Build history of the part. All positions in model axes, mm. A direction names the side the tool comes from. Give positions to 0.01 mm unless a question says otherwise; leave off trailing zeros. Order: outer loops, then holes, each group sorted by start corner. A loop starts at its lowest first (then second) coordinate and runs counter-clockwise, first axis right, second up. Notation, with made-up numbers: (58.5, -12.5) -> (66.5, -12.5) arc R12 ccw to (66.5, 0.5) -> close; hole circle Ø2 at (69.5, -32.5). An arc over 180 degrees is marked (long way). Write item = value, one per line. Start each with the question number.
Autodesk Inventor part; units mm, degrees
ref_plane "YZ Plane" through (0, 0, 0) normal (1, 0, 0) x (0, 1, 0)
ref_plane "XZ Plane" through (0, 0, 0) normal (0, 1, 0) x (-1, 0, 0)
ref_plane "XY Plane" through (0, 0, 0) normal (0, 0, 1) x (1, 0, 0)
sketch "Sketch1" plane through (0, 0, 0) normal (0, 0, 1) x (1, 0, 0)
  line L0 (51, -45) -> (-51, -45)
  line L1 (-51, -45) -> (-51, 45)
  line L2 (-51, 45) -> (51, 45)
  line L3 (51, 45) -> (51, -45)
  line L4 (51, -45) -> (-51, 45) construction
  line L5 (-51, -45) -> (51, 45) construction
  line L6 (-22, 0) -> (22, 0) construction
  line L7 (-36, 35) -> (-8, 35)
  line L8 (-8, 35) -> (-8, -35)
  line L9 (-8, -35) -> (-36, -35)
  line L10 (-36, -35) -> (-36, 35)
  line L11 (-36, 35) -> (-8, -35) construction
  line L12 (-8, 35) -> (-36, -35) construction
  line L13 (36, 35) -> (8, 35)
  line L14 (8, 35) -> (8, -35)
  line L15 (8, -35) -> (36, -35)
  line L16 (36, -35) -> (36, 35)
  line L17 (36, 35) -> (8, -35) construction
  line L18 (8, 35) -> (36, -35) construction
  point P0 (0, 0)
  point P1 (0, 0)
  dimension "d0" = 16
  dimension "d1" = 28
  dimension "d2" = 28
  dimension "d3" = 70
  dimension "d4" = 10
  dimension "d5" = 15
extrude "Extrusion1" add sketch "Sketch1" along normal blind 19
sketch "Sketch2" plane through (51, -45, 0) normal (1, 0, 0) x (0, 0, -1)
  circle A0 centre (0, 45) radius 7
  point P0 (0, 45)
  dimension "d8" = 14
extrude "Extrusion2" cut sketch "Sketch2" against normal through all
sketch "Sketch3" plane through (51, -45, 19) normal (1, 0, 0) x (0, 0, -1)
  arc A0 (19, 52) -> (19, 38) centre (19, 45) ccw
  circle A1 centre (19, 45) radius 18
  dimension "d11" = 36
extrude "Extrusion3" cut sketch "Sketch3" against normal blind 11
sketch "Sketch4" plane through (-51, -45, 19) normal (-1, 0, 0) x (0, 0, 1)
  arc A0 (-19, 38) -> (-19, 52) centre (-19, 45) ccw
  circle A1 centre (-19, 45) radius 17.5
  dimension "d14" = 35
extrude "Extrusion4" cut sketch "Sketch4" against normal blind 11
sketch "Sketch5" plane through (-8, -35, 19) normal (-1, 0, 0) x (0, 0, 1)
  arc A0 (-19, 28) -> (-19, 42) centre (-19, 35) ccw
  circle A1 centre (-19, 35) radius 17.5
  dimension "d17" = 35
extrude "Extrusion5" cut sketch "Sketch5" against normal blind 11
sketch "Sketch6" plane through (8, -35, 19) normal (1, 0, 0) x (0, 0, -1)
  arc A0 (19, 42) -> (19, 28) centre (19, 35) ccw
  circle A1 centre (19, 35) radius 17.5
  dimension "d20" = 35
extrude "Extrusion6" [suppressed]
sketch "Sketch7" plane through (0, 0, 19) normal (0, 0, 1) x (1, 0, 0)
  line L0 (-36, -35) -> (-36, 35)
  line L1 (-51, 45) -> (-51, -45)
  line L2 (0, 30) -> (0, -30) construction
  circle A0 centre (0, 30) radius 4
  circle A1 centre (0, -30) radius 4
  line L3 (43.5, -30) -> (-43.5, -30) construction
  line L4 (-43.5, -30) -> (-43.5, 30) construction
  line L5 (-43.5, 30) -> (43.5, 30) construction
  line L6 (43.5, 30) -> (43.5, -30) construction
  line L7 (43.5, -30) -> (-43.5, 30) construction
  line L8 (-43.5, -30) -> (43.5, 30) construction
  circle A2 centre (-43.5, 30) radius 4
  circle A3 centre (-43.5, -30) radius 4
  circle A4 centre (43.5, -30) radius 4
  circle A5 centre (43.5, 30) radius 4
  point P0 (0, 0)
  point P1 (0, 0)
  dimension "d23" = 60
  dimension "d24" = 8
  dimension "d25" = 7.5
  dimension "d26" = 87
extrude "Extrusion7" cut sketch "Sketch7" against normal through all
sketch "Sketch8" plane through (0, 0, 19) normal (0, 0, 1) x (1, 0, 0)
  line L0 (-51, 45) -> (-81, 45)
  line L1 (-81, 45) -> (-81, 31)
  line L2 (-81, 31) -> (-51, 31)
  line L3 (-51, 31) -> (-51, 45)
  line L4 (-51, -45) -> (-81, -45)
  line L5 (-81, -45) -> (-81, -31)
  line L6 (-81, -31) -> (-51, -31)
  line L7 (-51, -31) -> (-51, -45)
  line L8 (-81, 45) -> (-96, 45)
  line L9 (-96, 45) -> (-96, -45)
  line L10 (-96, -45) -> (-81, -45)
  line L11 (-81, -45) -> (-81, 45)
  point P0 (0, 0)
  dimension "d29" = 14
  dimension "d30" = 15
  dimension "d31" = 30
  dimension "d41" = 31
extrude "Extrusion8" add sketch "Sketch8" against normal up to surface (19 mm away)
sketch "Sketch9" plane through (-96, -45, 19) normal (-1, 0, 0) x (0, 0, 1)
  circle A0 centre (-19, 45) radius 17.5
  dimension "d34" = 35
extrude "Extrusion9" cut sketch "Sketch9" against normal blind 11
sketch "Sketch10" plane through (0, 0, 0) normal (0, 0, -1) x (-1, 0, 0)
  line L0 (96, -17.5) -> (85, -17.5)
  circle A0 centre (43.5, 30) radius 4
  circle A1 centre (0, 30) radius 4
  circle A2 centre (-43.5, 30) radius 4
  line L1 (85, 17.5) -> (96, 17.5)
  line L2 (96, 17.5) -> (96, 45)
  line L3 (96, 45) -> (-51, 45)
  line L4 (-51, 45) -> (-51, 18)
  line L5 (-51, 18) -> (-40, 18)
  line L6 (-40, 18) -> (-40, 7)
  line L7 (-40, 7) -> (-36, 7)
  line L8 (-36, 7) -> (-36, 35)
  line L9 (-36, 35) -> (-8, 35)
  line L10 (-8, -7) -> (-8, -35)
  line L11 (36, 7) -> (40, 7)
  line L12 (-3, 7) -> (-3, 17.5)
  line L13 (-3, 17.5) -> (8, 17.5)
  line L14 (8, 17.5) -> (8, 35)
  line L15 (8, 35) -> (36, 35)
  line L16 (36, 35) -> (36, 7)
  line L17 (40, 7) -> (40, 17.5)
  line L18 (40, 17.5) -> (51, 17.5)
  line L19 (51, 17.5) -> (51, 31)
  line L20 (51, 31) -> (81, 31)
  line L21 (81, 31) -> (81, -31)
  line L22 (90.5, 17.5) -> (90.5, 27.5) construction
  line L23 (91, -17.5) -> (91, -27.5) construction
  circle A3 centre (90.5, 27.5) radius 4
  circle A4 centre (91, -27.5) radius 4
  line L24 (96, -17.5) -> (85, -17.5)
  line L25 (81, -31) -> (51, -31)
  line L26 (51, -31) -> (51, -17.5)
  line L27 (51, -17.5) -> (40, -17.5)
  line L28 (40, -17.5) -> (40, -7)
  line L29 (40, -7) -> (36, -7)
  line L30 (36, -7) -> (36, -35)
  line L31 (36, -35) -> (8, -35)
  line L32 (8, -35) -> (8, -17.5)
  line L33 (8, -17.5) -> (-3, -17.5)
  line L34 (-3, -17.5) -> (-3, -7)
  line L35 (-3, -7) -> (-8, -7)
  line L36 (-8, -35) -> (-36, -35)
  line L37 (-36, -35) -> (-36, -7)
  line L38 (-36, -7) -> (-40, -7)
  line L39 (-40, -7) -> (-40, -18)
  line L40 (-40, -18) -> (-51, -18)
  line L41 (-51, -18) -> (-51, -45)
  line L42 (-51, -45) -> (96, -45)
  line L43 (96, -45) -> (96, -17.5)
  line L44 (-8, 35) -> (-8, 7)
  line L45 (-8, 7) -> (-3, 7)
  line L46 (85, -17.5) -> (85, 17.5)
  point P0 (86, -17.5)
  point P1 (0, 0)
  dimension "d37" = 8
  dimension "d38" = 10
extrude "Extrusion10" cut sketch "Sketch10" against normal through all contours A3 | A4
sketch "Sketch11" plane through (0, 0, 19) normal (0, 0, 1) x (1, 0, 0)
  circle A0 centre (-58.5, 38) radius 2.5
  circle A1 centre (-70.5, 38) radius 2.5
  circle A2 centre (-70.5, -38) radius 2.5
  circle A3 centre (-58.5, -38) radius 2.5
  point P0 (0, 0)
extrude "Extrusion11" cut sketch "Sketch11" against normal through all
sketch "Sketch12" plane through (-85, -45, 19) normal (-1, 0, 0) x (0, 0, 1)
  arc A0 (-19, 38) -> (-19, 52) centre (-19, 45) ccw
  line L0 (-19, 52) -> (-19, 38)
  line L1 (-19, 27.5) -> (-19, 62.5)
  point P0 (-19, 45)
extrude "Extrusion12" cut sketch "Sketch12" against normal blind 10
properties part number "frame 1"
(1) Cut at C-C, the plane x = -70.5. Give the cut face in (y, z), plus the area to 3 significant figures.
(2) Mould opens along Y. For faces 4 (the face through (-87.55, 30.2, 9.37)), 5 (the face through (-96, 1, 18)), 6 (the face through (36, 0, 9)), 7 (the face through (-21, -45, 9)) say: released by +Y, released by -Y, zero draft, split by the parting line, or undercut.
(3) Wall check: line 1 (X direction, y = -15, z = 13.5); line 2 (X direction, y = 7, z = 9); line 3 (Y direction, x = 30.5, z = 4). Give the ranges that are in metal, low to high. Write a range as [from, to].
(4) 3-axis set-ups, long thin cutter, end or side, ignore diameter. For faces 1 (the face through (-51, 0, 18)), 2 (the face through (46, 0, 18)), 3 (the face through (-2.577, -0.385, 17.496)): which of +Z, -Z, +X, -X, +Y, -Y reach the whole face in a straight line?
(5) Cut at D-D, the plane y = -27.5. Give the number of separate pieces and of enclosed holes in the cut face, plus the area to 3 significant figures.
(6) Cut at B-B, the plane x = 0. Give the cut face in (y, z).
(7) Flat gauge pins, fed straight in: P1, Ø5.5, axis at y = 5.5, z = 8, coming from the -X side; P2, Ø3, axis at x = -70.5, y = 38, coming from the -Z side; P3, Ø2, axis at y = 9.5, z = 12, coming from the +X side. Where does each tip first touch, or does it go through?
(8) Cut at A-A, the plane y = 38. Give the cut face in (x, z), plus the area to 3 significant figures.
Results:
q1.outline = (-45, 0) -> (-40.5, 0) -> (-40.5, 19) -> (-45, 19) -> close; (-35.5, 0) -> (-31, 0) -> (-31, 19) -> (-35.5, 19) -> close; (31, 0) -> (35.5, 0) -> (35.5, 19) -> (31, 19) -> close; (40.5, 0) -> (45, 0) -> (45, 19) -> (40.5, 19) -> close
q1.area = 342 mm2
q2.face_4 = undercut
q2.face_5 = zero draft
q2.face_6 = undercut
q2.face_7 = released by -Y
q3.line_1 = [-96, -81], [-51, -36], [-8, 8], [36, 51]
q3.line_2 = [-85, -81], [-40, -36], [3, 8], [36, 40]
q3.line_3 = [-45, -35], [35, 45]
q4.face_1 = +Z, -Z
q4.face_2 = -Z, +X
q4.face_3 = -Z
q5.separate_pieces = 8
q5.enclosed_holes = 0
q5.area = 651 mm2
q6.outline = (-45, 0) -> (-34, 0) -> (-34, 19) -> (-45, 19) -> close; (-26, 0) -> (-17.5, 0) arc R17.5 cw to (17.5, 0) -> (26, 0) -> (26, 19) -> (-26, 19) -> close; (34, 0) -> (45, 0) -> (45, 19) -> (34, 19) -> close
q7.P1 = -85
q7.P2 = through
q7.P3 = 40
q8.outline = (-96, 0) -> (-73, 0) -> (-73, 19) -> (-96, 19) -> close; (-68, 0) -> (-61, 0) -> (-61, 19) -> (-68, 19) -> close; (-56, 0) -> (51, 0) -> (51, 19) -> (-56, 19) -> close
q8.area = 2,600 mm2
